Job drawing, mm, ordinate dimensions from the low corner. One solid piece. Give positions to 0.01 mm unless a question says otherwise; leave off trailing zeros. Write each loop counter-clockwise with the first axis right and the second up, starting at its lowest first coordinate (ties: lowest second). Pieces come first, ordered by that corner, then holes. Notation, with made-up numbers: (32.25, 59.5) - (52.25, 59.5) arc R20 ccw to (52.25, 92.5) - close; hole circle Ø2 at (62, 64.5). An arc over 180 degrees is marked (long way). Answer as a JSON object with one key per item and string values.
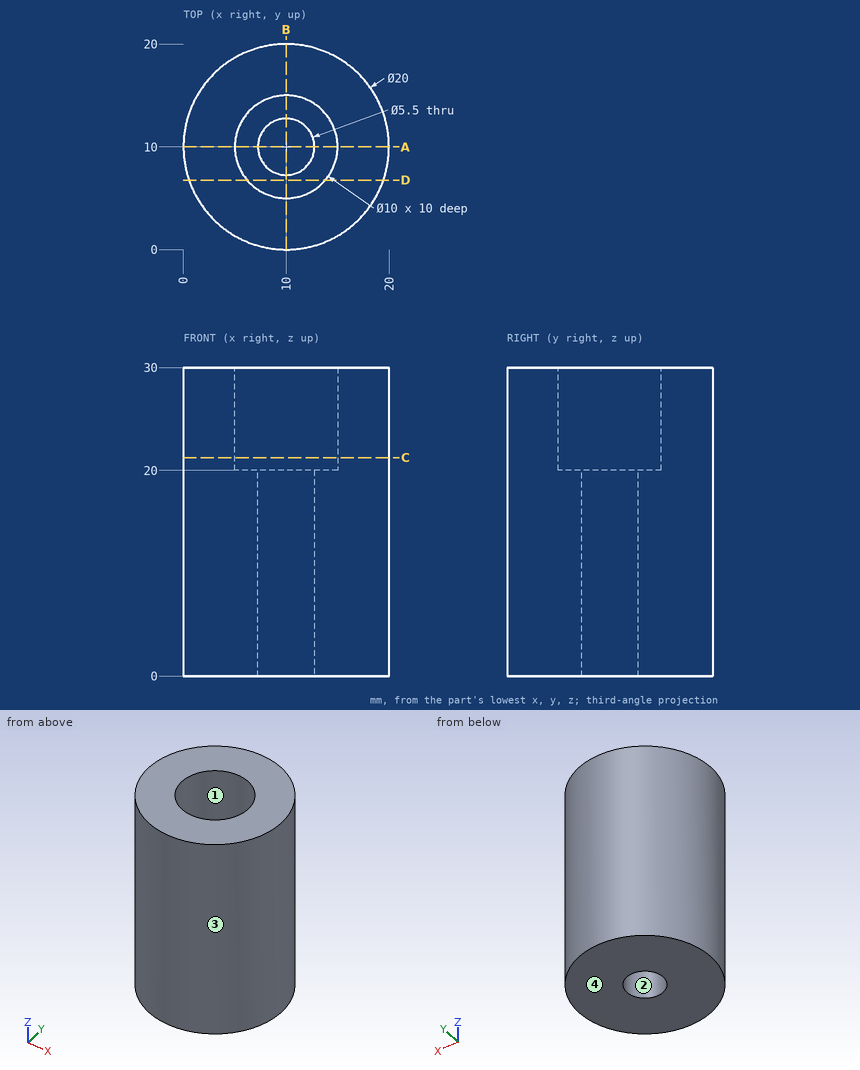
Item 1: Cut at A-A (y = 10). Give the cut face in (x, z).
Entries:
{"outline": "(0, 0) - (7.25, 0) - (7.25, 20) - (5, 20) - (5, 30) - (0, 30) - close; (12.75, 0) - (20, 0) - (20, 30) - (15, 30) - (15, 20) - (12.75, 20) - close"}
Item 2: Flat gauge pins, fed straight in: P1, Ø10, axis at x = 18, z = 14.5, coming from the +Y side; P2, Ø5, axis at y = 5, z = 26, coming from the +X side; P3, Ø8, axis at x = 3, z = 23.5, coming from the -Y side. Where does each tip first touch, or does it go through?
Entries:
{"P1": "y = 19.54", "P2": "x = 19.68", "P3": "y = 0.46"}
Item 3: Cut at C-C (z = 21.25). Give the cut face in (x, y).
Entries:
{"outline": "circle Ø20 at (10, 10); hole circle Ø10 at (10, 10)"}
Item 4: Probe line 1 (Y direction, x = 10, z = 7.5); line 2 (Y direction, x = 10, z = 23.5); line 3 (X direction, y = 6.75, z = 23.75). List the from-to ranges inside material, lowest first. Write a range as from..to.
Entries:
{"line 1": "0..7.25, 12.75..20", "line 2": "0..5, 15..20", "line 3": "0.54..6.2, 13.8..19.46"}
Item 5: Cut at D-D (y = 6.75). Give the cut face in (x, z), and give its area (3 significant figures).
Entries:
{"outline": "(0.54, 0) - (19.46, 0) - (19.46, 30) - (13.8, 30) - (13.8, 20) - (6.2, 20) - (6.2, 30) - (0.54, 30) - close", "area": "491 mm2"}
Item 6: Mould opens along Y. For the marked faces 1, 2, 3 and 4 say: +Y half, -Y half, draft (parallel to the pull), parting line (faces both ways), or undercut.
Entries:
{"face 1": "undercut", "face 2": "undercut", "face 3": "parting line", "face 4": "draft"}
